Input: part model. Units: mm. Frame: model coordinates. Face numbers are marked on the shaded views. A direction names the side the tool comes from. Round coordinates to 2 decimals unless told otherwise and drop trailing zeros. Order: outer loops, then holes, each group sorted by start corner. A loop starts at its lowest first (then second) coordinate and runs counter-clockwise, first axis right, second up. Notation, with made-up numbers: (-30.75, 64) -> (-16.75, 64) arc R21 cw to (-16.75, 98) -> close; hole circle Ø7 at (-16, 14.25). An arc over 180 degrees is marked (long way). Use a Markdown table: item, result.
from build123d import *

# Parameters (mm, degrees)
EXTRUDE_1_DEPTH          = 96
CUT_EXTRUDE_1_DEPTH      = 96
SKETCH_4_R               = 23.666666667
CUT_EXTRUDE_2_DEPTH      = 144
CUT_EXTRUDE_3_DEPTH      = 96
CUT_EXTRUDE_3_DEPTH_BACK = 96
SKETCH_7_R               = 9.192307692
CUT_EXTRUDE_4_DEPTH      = 20
SKETCH_8_R               = 6.666666667
EXTRUDE_2_DEPTH          = 3


with BuildPart() as part:
    # 草图1 → 旋转1 (revolve)
    with BuildSketch(Plane.XY, mode=Mode.PRIVATE) as revolve_1_sk:
        Polygon((0, -18), (24.666666667, -18), (24.666666667, -20), (26.666666667, -20), (26.666666667, -162), (0, -162), align=None)
    revolve(revolve_1_sk.sketch.rotate(Axis((0, -162, 0), (0, 1, 0)), 270), axis=Axis((0, -162, 0), (0, 1, 0)))

    # 草图2 → 凸台-拉伸1 (add)
    with BuildSketch(Plane.XY):
        with BuildLine():
            Line((-22, -171), (-19, -171))
            Line((-19, -171), (-19, -31))
            ThreePointArc((-19, -31), (-18.707106781, -30.292893219), (-18, -30))
            Line((-18, -30), (18, -30))
            ThreePointArc((18, -30), (18.707106781, -30.292893219), (19, -31))
            Line((19, -31), (19, -171))
            Line((19, -171), (22, -171))
            Line((22, -171), (22, -30))
            ThreePointArc((22, -30), (21.121320344, -27.878679656), (19, -27))
            Line((19, -27), (-19, -27))
            ThreePointArc((-19, -27), (-21.121320344, -27.878679656), (-22, -30))
            Line((-22, -30), (-22, -171))
        make_face()
    extrude(amount=EXTRUDE_1_DEPTH)

    # 草图3 → 切除-拉伸1 (cut)
    with BuildSketch(Plane.XY):
        with BuildLine():
            Line((-19, -171), (19, -171))
            Line((19, -171), (19, -31))
            ThreePointArc((19, -31), (18.707106781, -30.292893219), (18, -30))
            Line((18, -30), (-18, -30))
            ThreePointArc((-18, -30), (-18.707106781, -30.292893219), (-19, -31))
            Line((-19, -31), (-19, -171))
        make_face()
    extrude(amount=CUT_EXTRUDE_1_DEPTH, mode=Mode.SUBTRACT)

    # 草图4 → 切除-拉伸2 (cut)
    with BuildSketch(Plane(origin=(0, -21, 0), x_dir=(1, 0, 0), z_dir=(0, 1, 0))):
        with Locations(Location((0, 0, 0), (0, 0, 270))):
            Circle(SKETCH_4_R)
    extrude(amount=-CUT_EXTRUDE_2_DEPTH, mode=Mode.SUBTRACT)

    # 草图5 → 切除-拉伸3 (cut, two sides: drawn at the far end of the back side and taken through both)
    with BuildSketch(Plane(origin=(0, 0, 0), x_dir=(0, 0, -1), z_dir=(1, 0, 0)).offset(-CUT_EXTRUDE_3_DEPTH_BACK)):
        with BuildLine():
            Line((-150, -250), (50, -250))
            Line((50, -250), (50, -27))
            Line((50, -27), (25.585063646, -27))
            ThreePointArc((25.585063646, -27), (22.304312848, -27.976388331), (20.091324315, -30.587775267))
            Line((20.091324315, -30.587775267), (-14.545091957, -109.470741578))
            ThreePointArc((-14.545091957, -109.470741578), (-15.282754801, -110.34120389), (-16.3763384, -110.666666667))
            Line((-16.3763384, -110.666666667), (-35, -110.666666667))
            ThreePointArc((-35, -110.666666667), (-46.78511302, -105.78511302), (-51.666666667, -94))
            Line((-51.666666667, -94), (-51.666666667, 0))
            Line((-51.666666667, 0), (-150, 0))
            Line((-150, 0), (-150, -250))
        make_face()
    extrude(amount=CUT_EXTRUDE_3_DEPTH + CUT_EXTRUDE_3_DEPTH_BACK, mode=Mode.SUBTRACT)

    # 草图6 → 旋转2 (revolve)
    with BuildSketch(Plane.XY.offset(35), mode=Mode.PRIVATE) as revolve_2_sk:
        with BuildLine():
            Line((-34, -94), (-34, -90.602564103))
            Line((-34, -90.602564103), (-33.230769231, -89.833333333))
            Line((-33.230769231, -89.833333333), (-30, -89.833333333))
            ThreePointArc((-30, -89.833333333), (-29.556324994, -87.639723002), (-28.5, -85.666666667))
            Line((-28.5, -85.666666667), (-22, -85.666666667))
            Line((-22, -85.666666667), (-22, -94))
            Line((-22, -94), (-34, -94))
        make_face()
    revolve(revolve_2_sk.sketch.rotate(Axis((-22, -94, 35), (-1, 0, 0)), 270), axis=Axis((-22, -94, 35), (-1, 0, 0)))

    # 草图7 → 切除-拉伸4 (cut)
    with BuildSketch(Plane(origin=(-22, 0, 0), x_dir=(0, 0, -1), z_dir=(1, 0, 0))):
        with Locations((-35, -94)):
            Circle(SKETCH_7_R)
        Polygon((-42.142857143, -89.876069506), (-42.142857143, -98.123930494), (-35, -102.247860988), (-27.857142857, -98.123930494), (-27.857142857, -89.876069506), (-35, -85.752139012), align=None, mode=Mode.SUBTRACT)
    extrude(amount=-CUT_EXTRUDE_4_DEPTH, mode=Mode.SUBTRACT)

    # 草图8 → 凸台-拉伸2 (add)
    with BuildSketch(Plane(origin=(22, 0, 0), x_dir=(0, 0, -1), z_dir=(1, 0, 0))):
        with Locations(Location((-35, -94, 0), (0, 0, 180))):
            Circle(SKETCH_8_R)
    extrude(amount=EXTRUDE_2_DEPTH)


solid = part.part
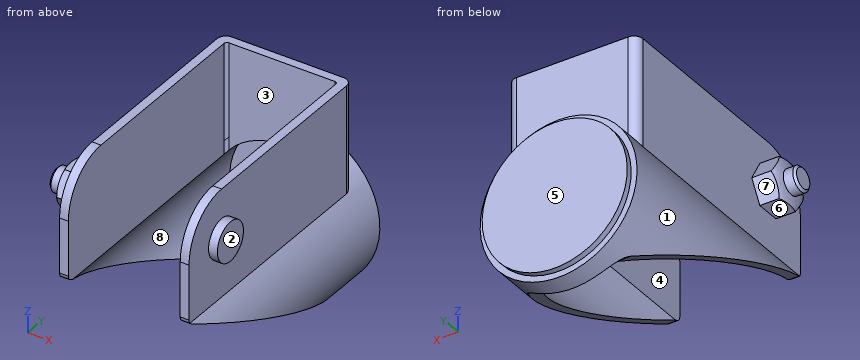
1) Pin query (flat end, axial travel): pin 1 Ø4 at (x, z) = (-9.5, 41) entering from +Y; pin 2 Ø12 at (x, y) = (18.5, -49.5) entering from +Z; pin 3 Ø4 at (x, y) = (-15.5, -77) entering from -Z; pin 4 Ø23.5 at (x, z) = (0.5, 5) entering from -Y. Return the tip coordinate at first contact, or that it passes through.
Results found:
| item | result |
|---|---|
| pin 1 | stops at y = -27 |
| pin 2 | stops at z = 51.67 |
| pin 3 | passes through |
| pin 4 | stops at y = -21 |
2) Cut plane A-A on y = -77. Return loops of the section in (x, z).
Results found:
| item | result |
|---|---|
| outline | (-26.67, 0.29) -> (-23.66, 0.29) arc R23.67 cw to (-19, 14.11) -> (-19, 51.67) -> (-22, 51.67) -> (-22, 15.07) arc R26.67 ccw to start; (19, 14.11) arc R23.67 cw to (23.66, 0.29) -> (26.67, 0.29) arc R26.67 ccw to (22, 15.07) -> (22, 51.67) -> (19, 51.67) -> close |
3) Cut plane B-B on z = -19. Return loops of the section in (x, y).
Results found:
| item | result |
|---|---|
| outline | (-18.71, -33.07) -> (-14.11, -33.07) -> (-14.11, -21) -> (14.11, -21) -> (14.11, -33.07) -> (18.71, -33.07) -> (18.71, -20) -> (15.73, -20) -> (15.73, -18) -> (-15.73, -18) -> (-15.73, -20) -> (-18.71, -20) -> close |
4) Line query: L1, parallel to X at y = -92.5, z = 22; L2, parallel to X at y = -60.5, z = 0; L3, parallel to Y at x = -10.5, z = 30. Output: solid intervals per line, ascending. Write a range as [from, to].
Results found:
| item | result |
|---|---|
| L1 | x = [-22, -19], [19, 22] |
| L2 | x = [-26.67, -23.67], [23.67, 26.67] |
| L3 | y = [-30, -27] |
5) Pull-direction query (X, two-part tool) for the marked faces 1, 2, 3 and 4; classes: +X half, -X half, draft (parallel to the pull), parting line (faces both ways), or undercut.
Results found:
| item | result |
|---|---|
| face 1 | parting line |
| face 2 | +X half |
| face 3 | undercut |
| face 4 | undercut |
6) Cut plane D-D on y = -39.5. Return loops of the section in (x, z).
Results found:
| item | result |
|---|---|
| outline | (-22, 15.07) arc R26.67 ccw to (-21.2, -16.18) -> (-17.27, -16.18) arc R23.67 cw to (-19, 14.11) -> (-19, 51.67) -> (-22, 51.67) -> close; (17.27, -16.18) -> (21.2, -16.18) arc R26.67 ccw to (22, 15.07) -> (22, 51.67) -> (19, 51.67) -> (19, 14.11) arc R23.67 cw to start |
7) Cut plane C-C on x = -15. Return loops of the section in (y, z).
Results found:
| item | result |
|---|---|
| outline | (-34.65, -18.31) -> (-30.59, -20.09) arc R6 cw to (-28.15, -22.05) -> (-20, -22.05) -> (-20, -19.58) -> (-18, -19.58) -> (-18, 19.58) -> (-20, 19.58) -> (-20, 22.05) -> (-27, 22.05) -> (-27, 51.67) -> (-30, 51.67) -> (-30, 18.31) -> (-21, 18.31) -> (-21, -18.31) -> close |
8) Set-up query: the marked faces 5, 6, 7 and 8. Return all of +Z, -Z, +X, -X, +Y, -Y with unobstructed straight access to the full face (end or side cutting, diameter ignored); none if empty.
Results found:
| item | result |
|---|---|
| face 5 | +Z, -Z, +X, -X, +Y |
| face 6 | -X, +Y, -Y |
| face 7 | -X, +Y |
| face 8 | -Y |
